Build history of the part. All positions in model axes, mm. A direction names the side the tool comes from. Round coordinates to 2 decimals unless told otherwise and drop trailing zeros. Loops run counter-clockwise (first coordinate to the right, second up) from the corner with the lowest first, then second, coordinate; pieces in that order, holes last.
from build123d import *

# Parameters (mm, degrees)
SZKIC1_W                    = 250
SZKIC1_H                    = 250
DODANIE_WYCI_GNI_CIE1_DEPTH = 300
SZKIC2_W                    = 240
SZKIC2_H                    = 240
WYTNIJ_WYCI_GNI_CIE1_DEPTH  = 295
SZKIC3_W                    = 240
SZKIC3_H                    = 240
SZKIC3_W_2                  = 200
SZKIC3_H_2                  = 200
DODANIE_WYCI_GNI_CIE2_DEPTH = 20


with BuildPart() as part:
    # Szkic1 → Dodanie-wyciągnięcie1 (new body)
    with BuildSketch(Plane(origin=(0, 0, 0), x_dir=(1, 0, 0), z_dir=(0, 1, 0))):
        with Locations((-34.375, -85.9375)):
            Rectangle(SZKIC1_W, SZKIC1_H)
    extrude(amount=DODANIE_WYCI_GNI_CIE1_DEPTH)

    # Szkic2 → Wytnij-wyciągnięcie1 (cut)
    with BuildSketch(Plane(origin=(0, 300, 0), x_dir=(1, 0, 0), z_dir=(0, 1, 0))):
        with Locations((-34.375, -85.9375)):
            Rectangle(SZKIC2_W, SZKIC2_H)
    extrude(amount=-WYTNIJ_WYCI_GNI_CIE1_DEPTH, mode=Mode.SUBTRACT)

    # Szkic3 → Dodanie-wyciągnięcie2 (add)
    with BuildSketch(Plane(origin=(0, 300, 0), x_dir=(1, 0, 0), z_dir=(0, 1, 0))):
        with Locations((-34.375, -85.9375)):
            Rectangle(SZKIC3_W, SZKIC3_H)
        with Locations((-34.375, -85.9375)):
            Rectangle(SZKIC3_W_2, SZKIC3_H_2, mode=Mode.SUBTRACT)
    extrude(amount=-DODANIE_WYCI_GNI_CIE2_DEPTH)


solid = part.part
(1) Pin check, flat tip, straight feed: P1, Ø4, axis at x = -38.5, z = 115, coming from the +Y side. Stop position of the tip, or through.
Responses:
P1: stops at y = 5
(2) Slice it at A-A on y = 52.5. List the corners of the cut face in (x, z) (1 decimal).
Responses:
outline: (-159.4, -39.1) - (90.6, -39.1) - (90.6, 210.9) - (-159.4, 210.9) - close; hole (-154.4, -34.1) - (85.6, -34.1) - (85.6, 205.9) - (-154.4, 205.9) - close
(3) Slice it at B-B on z = 12. List the corners of the cut face in (x, y) (3 decimals).
Responses:
outline: (-159.375, 0) - (90.625, 0) - (90.625, 300) - (65.625, 300) - (65.625, 280) - (85.625, 280) - (85.625, 5) - (-154.375, 5) - (-154.375, 280) - (-134.375, 280) - (-134.375, 300) - (-159.375, 300) - close
(4) Probe line 1 (Y direction, x = -82, z = 188.5); line 2 (Z direction, x = -42.5, y = 38); line 3 (X direction, y = 70, z = -14.5) (3 decimals). List the from-to ranges inside material, lowest first.
Responses:
line 1: y = 0 to 5, 280 to 300
line 2: z = -39.06 to -34.06, 205.94 to 210.94
line 3: x = -159.375 to -154.375, 85.625 to 90.625
(5) Pull direction Y, two halves, no side cores. Call faces 4 (the face through (-154.375, 144, 88)), 5 (the face through (-36, 0, 84)), 6 (the face through (-159.375, 148, 88)), 7 (the face through (-147, 300, 84)): +Y half, -Y half, draft (parallel to the pull), parting line (faces both ways), or undercut.
Responses:
face 4: undercut
face 5: -Y half
face 6: draft
face 7: +Y half
(6) Slice it at C-C on x = -11. List the corners of the cut face in (y, z).
Responses:
outline: (0, -39.06) - (300, -39.06) - (300, -14.06) - (280, -14.06) - (280, -34.06) - (5, -34.06) - (5, 205.94) - (280, 205.94) - (280, 185.94) - (300, 185.94) - (300, 210.94) - (0, 210.94) - close
(7) Which spindle directions (+Z, -Z, +X, -X, +Y, -Y) get a long thin tool onto all of the face, cutting with end or side? Do faces 1 (the face through (-36, 144, 205.938)), 2 (the face through (65.625, 290, 87)), 3 (the face through (-36, 148, 210.938)). Say none if no direction does.
Responses:
face 1: none
face 2: +Y
face 3: +Z, +X, -X, +Y, -Y
